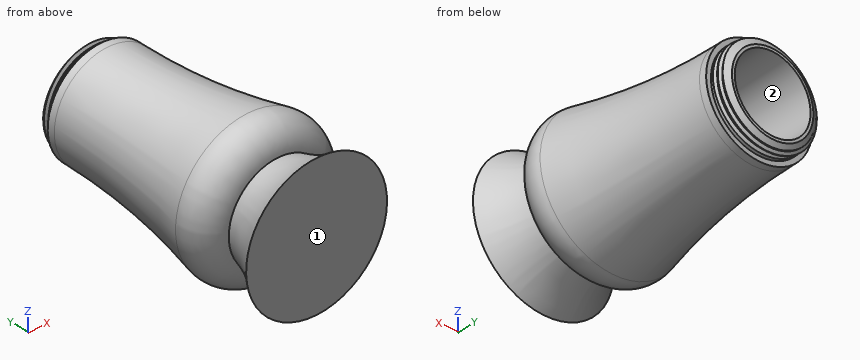
from build123d import *
from build123d.topology import SkipClean

# Parameters (mm, degrees)
GWINT1_PITCH               = 1
SZKIC10_R                  = 7
WYTNIJ_WYCI_GNI_CIE2_DEPTH = 25
ZAOKR_GLENIE1_R            = 5


with BuildPart() as part:
    # Szkic2 → Obrót1 (revolve)
    with BuildSketch(Plane.XY, mode=Mode.PRIVATE) as obr_t1_sk:
        with BuildLine():
            Line((0, 0), (0, 8))
            Line((0, 8), (9.027373354, 8))
            ThreePointArc((9.027373354, 8), (10.570833484, 3.780088701), (13, 0))
            Line((13, 0), (0, 0))
        make_face()
    revolve(obr_t1_sk.sketch.rotate(Axis((0, 0, 0), (0, 1, 0)), 90), axis=Axis((0, 0, 0), (0, 1, 0)))

    # Szkic4 → Obrót2 (revolve)
    with BuildSketch(Plane.XY, mode=Mode.PRIVATE) as obr_t2_sk:
        with BuildLine():
            Line((0, 8), (0, 43))
            Line((0, 43), (0, 47.12232406))
            Line((0, 47.12232406), (8.9, 47.12232406))
            Line((8.9, 47.12232406), (8.9, 45.06116203))
            Line((8.9, 45.06116203), (8.9, 44.597825987))
            Line((8.9, 44.597825987), (8.9, 44.463010207))
            Line((8.9, 44.463010207), (8.9, 44.359094252))
            Line((8.9, 44.359094252), (9.8, 44.359094252))
            Line((9.8, 44.359094252), (9.8, 43))
            ThreePointArc((9.8, 43), (11.129787622, 25.311282732), (15, 8))
            Line((15, 8), (0, 8))
        make_face()
    revolve(obr_t2_sk.sketch.rotate(Axis((0, 8, 0), (0, 1, 0)), 90), axis=Axis((0, 8, 0), (0, 1, 0)))

    # Gwint1: the profile of Profil gwintu1 profile screwed along a right-hand helix of 2 turns, 8 arcs to a turn; built about Z, then put on its axis
    with SkipClean():  # the faces are left unmerged after this step: merging them gives an invalid solid
        gwint1_z = Axis((0, 0, 0), (0, 0, 1))
        gwint1_corners = [(8.9003, 0, -0.000173205), (8.9003, 0, 0.875173202), (8.358734125, 0, 0.562499998), (8.358734125, 0, 0.312499998)]
        with BuildLine(mode=Mode.PRIVATE) as gwint1_profile:
            Line(gwint1_corners[0], gwint1_corners[1])
            Line(gwint1_corners[1], gwint1_corners[2])
            Line(gwint1_corners[2], gwint1_corners[3])
            Line(gwint1_corners[3], gwint1_corners[0])
        gwint1_cap = Face(gwint1_profile.wire())
        gwint1_turn_angles = [0, 22.5, 45, 67.5, 90, 112.5, 135, 157.5, 180, 202.5, 225, 247.5, 270, 292.5, 315, 337.5, 360]
        gwint1_turn_weights = [1, 0.9238795325112867, 1, 0.9238795325112867, 1, 0.9238795325112867, 1, 0.9238795325112867, 1, 0.9238795325112867, 1, 0.9238795325112867, 1, 0.9238795325112867, 1, 0.9238795325112867, 1]
        gwint1_turn_rails = [Edge.make_bspline([Vector(p[0], p[1], 0).rotate(gwint1_z, gwint1_turn_angles[k]) / gwint1_turn_weights[k] + Vector(0, 0, p[2] + GWINT1_PITCH * gwint1_turn_angles[k] / 360) for k in range(17)], [0, 0, 0, 1, 1, 2, 2, 3, 3, 4, 4, 5, 5, 6, 6, 7, 7, 8, 8, 8], 2, gwint1_turn_weights) for p in gwint1_corners]
        gwint1_turn_sides = [Face.make_surface_from_curves(gwint1_turn_rails[p[0]], gwint1_turn_rails[p[1]]) for p in [(0, 1), (1, 2), (2, 3), (3, 0)]]
        gwint1 = Plane(origin=(0, 47.12232406, 0), x_dir=(-1, 0, 0), z_dir=(0, -1, 0)) * Solid(Shell([*[p.moved(Location((0, 0, GWINT1_PITCH * i))) for i in range(2) for p in gwint1_turn_sides], gwint1_cap, gwint1_cap.rotate(gwint1_z, 720).moved(Location((0, 0, GWINT1_PITCH * 720 / 360)))]))
        add(gwint1, mode=Mode.SUBTRACT)

    # Wycięcie-wyciągnięcie po ścieżce1: sweep along a path in Szkic8
    with BuildLine(Plane(origin=(0, 47.12232406, 0), x_dir=(1, 0, 0), z_dir=(0, 1, 0))) as wyci_cie_wyci_gni_cie_po_cie_ce1_path:
        CenterArc((0, 0), 13, 0, 360)
    # Szkic9 → Wycięcie-wyciągnięcie po ścieżce1 (sweep, cut)
    with BuildSketch(Plane.XY):
        Polygon((8.9, 47.12232406), (8.9, 46.32232406), (7.514359354, 47.12232406), align=None)
    sweep(path=wyci_cie_wyci_gni_cie_po_cie_ce1_path.line, mode=Mode.SUBTRACT)

    # Szkic10 → Wytnij-wyciągnięcie2 (cut)
    with BuildSketch(Plane(origin=(0, 47.12232406, 0), x_dir=(1, 0, 0), z_dir=(0, 1, 0))):
        with Locations(Location((0, 0, 0), (0, 0, 270))):
            Circle(SZKIC10_R)
    extrude(amount=-WYTNIJ_WYCI_GNI_CIE2_DEPTH, mode=Mode.SUBTRACT)

    # Zaokrąglenie1
    # the kernel refuses this fillet: 5 mm, written as the material it takes off along each edge
    with BuildSketch(Plane(origin=(0, 8, 0), x_dir=(0, 0, -1), z_dir=(1, 0, 0))) as zaokr_glenie1_piece_1:
        with BuildLine():
            CenterArc((8.463528587, 4.968106186), ZAOKR_GLENIE1_R, 276.47495836, 97.293161414)
            Line((9.027373354, 0), (15, 0))
            ThreePointArc((15, 0), (14.119819715, 3.068091884), (13.319862852, 6.158071522))
        make_face()
    revolve(axis=Axis((0, 8, 0), (0, 1, 0)), mode=Mode.SUBTRACT)


solid = part.part
Could you check a few things on this model? Use its own coordinates, in mm. Face numbers are marked on the shaded views. Round coordinates to 2 decimals unless told otherwise and drop trailing zeros. Write each loop counter-clockwise with the first axis right and the second up, starting at its lowest first coordinate (ties: lowest second). Pieces come first, ordered by that corner, then holes. Notation, with made-up numbers: (46, 45) -> (58, 45) arc R21 ccw to (58, 57) -> close; hole circle Ø10 at (-23.5, -28). An arc over 180 degrees is marked (long way). Use a Markdown table: item, result.
1. For pin 1 Ø1.5 at (y, z) = (18, -2) entering from -X; pin 2 Ø1.5 at (x, y) = (10.5, 26.5) entering from -Z; pin 3 Ø6 at (x, z) = (-1, -2) entering from +Y, each with a flat end and sliding along its axis, tell me the tip position at first contact or that it passes through.
Answer key:
| item | result |
|---|---|
| pin 1 | stops at x = -12.48 |
| pin 2 | stops at z = -5.02 |
| pin 3 | stops at y = 22.12 |
2. Please list where these lines run through material, in increasing order: probe 1 along X at (y, z) = (42.25, 0); probe 2 along Z at (x, y) = (3.5, 22.5); probe 3 along X at (y, z) = (35.5, 0).
Answer key:
| item | result |
|---|---|
| probe 1 | x = -9.8 to -7, 7 to 9.8 |
| probe 2 | z = -11.04 to -6.06, 6.06 to 11.04 |
| probe 3 | x = -10.05 to -7, 7 to 10.05 |
3. We'd pull the mould along Z, two halves only. Please class the marked faces 1 and 2: +Z half, -Z half, draft (parallel to the pull), parting line (faces both ways), or undercut.
Answer key:
| item | result |
|---|---|
| face 1 | draft |
| face 2 | undercut |
4. If we section it at B-B (y = 11): List the corners of the cut face in (x, z) for me.
Answer key:
| item | result |
|---|---|
| outline | circle Ø26.12 at (0, 0) |
5. If we section it at A-A (y = 30): List the corners of the cut face in (x, z) for me, then the cut area to 3 significant figures.
Answer key:
| item | result |
|---|---|
| outline | circle Ø21.05 at (0, 0); hole circle Ø14 at (0, 0) |
| area | 194 mm^2 |
